Study the drawing (mm; zero at the part's minimum x, y, z) and answer. A direction names the side the tool comes from. Round coordinates to 2 decimals unless told otherwise and drop trailing zeros. Order: outer loops, then holes, each group sorted by start corner. A loop starts at its lowest first (then second) coordinate and runs counter-clockwise, first axis right, second up. Notation, with made-up numbers: (4, -39.5) -> (47, -39.5) arc R14 ccw to (47, -17.5) -> close; hole circle Ø2 at (34.25, 70.5). An arc over 180 degrees is marked (long way). Use one line per item in the form item = value.
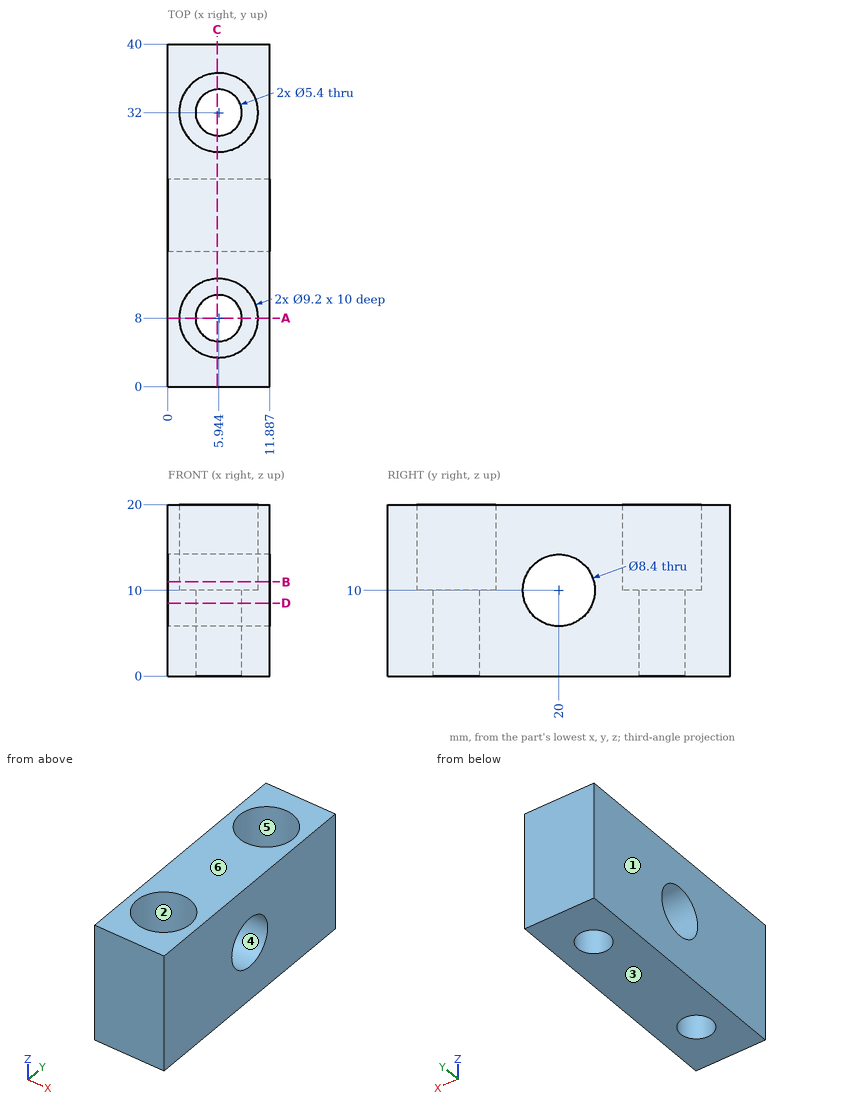
Item 1: The part is cut by section B-B, the plane z = 11. Give the vertices of the cut face in (x, y).
Findings:
outline = (0, 0) -> (11.89, 0) -> (11.89, 15.92) -> (0, 15.92) -> close; (0, 24.08) -> (11.89, 24.08) -> (11.89, 40) -> (0, 40) -> close; hole circle Ø9.2 at (5.94, 8); hole circle Ø9.2 at (5.94, 32)
Item 2: For the marked faces 1 and 2, determine the directions among +Z, -Z, +X, -X, +Y, -Y from which every point of the face is accessible in a straight line to the end or side of a thin tool.
Findings:
face_1 = +Z, -Z, -X, +Y, -Y
face_2 = +Z
Item 3: Determine the mould class of the marked faces 3, 4, 5 and 6 for opening direction Z: released by +Z, released by -Z, zero draft, split by the parting line, or undercut.
Findings:
face_3 = released by -Z
face_4 = undercut
face_5 = zero draft
face_6 = released by +Z
Item 4: A flat-ended cylindrical pin translates along its axis: P1, Ø1.5, axis at x = 5.5, y = 34, coming from the +Z side. Find the tip coordinate at first contact, or state that the pin passes through.
Findings:
P1 = 10
Item 5: The part is cut by section C-C, the plane x = 5.75. Give the vertices of the cut face in (y, z), and give its area (3 significant figures).
Findings:
outline = (0, 0) -> (5.31, 0) -> (5.31, 10) -> (3.4, 10) -> (3.4, 20) -> (0, 20) -> close; (10.69, 0) -> (29.31, 0) -> (29.31, 10) -> (27.4, 10) -> (27.4, 20) -> (12.6, 20) -> (12.6, 10) -> (10.69, 10) -> close; (34.69, 0) -> (40, 0) -> (40, 20) -> (36.6, 20) -> (36.6, 10) -> (34.69, 10) -> close; hole circle Ø8.4 at (20, 10)
area = 453 mm^2
Item 6: Consider line 1 along Y through (x, z) = (7.25, 8.5); line 2 along Y through (x, z) = (2.5, 15.5); line 3 along Y through (x, z) = (2, 18.75) (1 decimal). Determine where each line is inside the solid, lowest interval first.
Findings:
line_1 = 0 to 5.64, 10.36 to 16.08, 23.92 to 29.64, 34.36 to 40
line_2 = 0 to 4.95, 11.05 to 28.95, 35.05 to 40
line_3 = 0 to 5.6, 10.4 to 29.6, 34.4 to 40
Item 7: The part is cut by section A-A, the plane y = 8. Give the vertices of the cut face in (x, z).
Findings:
outline = (0, 0) -> (3.24, 0) -> (3.24, 10) -> (1.34, 10) -> (1.34, 20) -> (0, 20) -> close; (8.64, 0) -> (11.89, 0) -> (11.89, 20) -> (10.54, 20) -> (10.54, 10) -> (8.64, 10) -> close
Item 8: The part is cut by section D-D, the plane z = 8.5. Give the vertices of the cut face in (x, y).
Findings:
outline = (0, 0) -> (11.89, 0) -> (11.89, 16.08) -> (0, 16.08) -> close; (0, 23.92) -> (11.89, 23.92) -> (11.89, 40) -> (0, 40) -> close; hole circle Ø5.4 at (5.94, 8); hole circle Ø5.4 at (5.94, 32)
